Part model, mm, in its own coordinate system. A direction names the side the tool comes from. Coordinates: 2 decimals unless noted, no trailing zeros. Order: outer loops, then holes, each group sorted by start corner. A loop starts at its lowest first (then second) coordinate and runs counter-clockwise, first axis right, second up. Notation, with made-up numbers: M -13,65 L -2,65 A20 ccw -2,78 Z; hole C 87.25,37.25 d2. An arc over 180 degrees is marked long. Write item = value, one per line. Start each with the question number.
from build123d import *

# Parameters (mm, degrees)
SKETCH_1_W          = 23
SKETCH_1_H          = 23
EXTRUDE_1_DEPTH     = 1.6
SKETCH_2_W          = 5
SKETCH_2_H          = 4
EXTRUDE_2_DEPTH     = 1.6
FILLET_1_R          = 4
CUT_EXTRUDE_1_REACH = 18.575
SKETCH_3_R          = 1.6


with BuildPart() as part:
    # 草图1 → 凸台-拉伸1 (new body)
    with BuildSketch(Plane(origin=(0, 0, 0), x_dir=(1, 0, 0), z_dir=(0, 1, 0))):
        Rectangle(SKETCH_1_W, SKETCH_1_H)
    extrude(amount=EXTRUDE_1_DEPTH)

    # 草图2 → 凸台-拉伸2 (add)
    with BuildSketch(Plane(origin=(0, 1.6, 0), x_dir=(1, 0, 0), z_dir=(0, 1, 0))):
        Rectangle(SKETCH_2_W, SKETCH_2_H)
    extrude(amount=EXTRUDE_2_DEPTH)

    # 圆角1
    fillet_1_edges = [part.edges().sort_by_distance(p)[0] for p in [
        (11.5, 0.8, 11.5),
        (-11.5, 0.8, 11.5),
        (-11.5, 0.8, -11.5),
        (11.5, 0.8, -11.5),
    ]]
    fillet(fillet_1_edges, radius=FILLET_1_R)

    # 草图3 → 切除-拉伸1 (cut, up to next)
    with BuildSketch(Plane.XZ, mode=Mode.PRIVATE) as cut_extrude_1_sk1:
        with Locations(Location((-8, 8, 0), (0, 0, 270))):
            Circle(SKETCH_3_R)
    cut_extrude_1_tool1 = extrude(cut_extrude_1_sk1.sketch, amount=-CUT_EXTRUDE_1_REACH, mode=Mode.PRIVATE) & part.part
    # 草图3 → 切除-拉伸1 (cut, up to next)
    with BuildSketch(Plane.XZ, mode=Mode.PRIVATE) as cut_extrude_1_sk2:
        with Locations(Location((8, 8, 0), (0, 0, 270))):
            Circle(SKETCH_3_R)
    cut_extrude_1_tool2 = extrude(cut_extrude_1_sk2.sketch, amount=-CUT_EXTRUDE_1_REACH, mode=Mode.PRIVATE) & part.part
    # 草图3 → 切除-拉伸1 (cut, up to next)
    with BuildSketch(Plane.XZ, mode=Mode.PRIVATE) as cut_extrude_1_sk3:
        with Locations(Location((8, -8, 0), (0, 0, 270))):
            Circle(SKETCH_3_R)
    cut_extrude_1_tool3 = extrude(cut_extrude_1_sk3.sketch, amount=-CUT_EXTRUDE_1_REACH, mode=Mode.PRIVATE) & part.part
    # 草图3 → 切除-拉伸1 (cut, up to next)
    with BuildSketch(Plane.XZ, mode=Mode.PRIVATE) as cut_extrude_1_sk4:
        with Locations(Location((-8, -8, 0), (0, 0, 270))):
            Circle(SKETCH_3_R)
    cut_extrude_1_tool4 = extrude(cut_extrude_1_sk4.sketch, amount=-CUT_EXTRUDE_1_REACH, mode=Mode.PRIVATE) & part.part
    add(cut_extrude_1_tool1.solids().sort_by_distance((-8, 0, 8))[0], mode=Mode.SUBTRACT)
    add(cut_extrude_1_tool2.solids().sort_by_distance((8, 0, 8))[0], mode=Mode.SUBTRACT)
    add(cut_extrude_1_tool3.solids().sort_by_distance((8, 0, -8))[0], mode=Mode.SUBTRACT)
    add(cut_extrude_1_tool4.solids().sort_by_distance((-8, 0, -8))[0], mode=Mode.SUBTRACT)


solid = part.part
Item 1: Flat gauge pins, fed straight in: pin 1 (4 mm diameter, centred on x = -8, z = 8, fed in from +Y); pin 2 (2.5 mm diameter, centred on x = -8, z = -8, fed in from +Y); pin 3 (0.5 mm diameter, centred on x = 0, y = 3, fed in from -Z); pin 4 (0.5 mm diameter, centred on y = 2.5, z = 0, fed in from -X). Where does each tip first touch, or does it go through?
Item 2: Cut at B-B, the plane z = -8. Write the cut outline in (x, y).
Item 3: Wall check: line 1 along X through (y, z) = (0.4, -8); line 2 along Y through (x, z) = (1.5, -10); line 3 along X through (y, z) = (2.45, 0.5). Give the ranges that are in metal, low to high. Write a range as [from, to].
Item 4: Cut at C-C, the plane x = -1.5. Write the cut outline in (y, z), and give its area (3 significant figures).
Item 5: Cut at D-D, the plane x = -8. Write the cut outline in (y, z).
Item 6: Pull direction X, two halves, no side cores. Call faces 1 (the flat face through (-0.2, 1.6, 2.4)), 2 (the cylindrical face through (7.03, 0.79, 9.27)), 3 (the cylindrical face through (10.297, 0.811, -10.359)): pulls with the +X half, pulls with the -X half, needs draft (parallel to the pull), parting line crosses it, or undercut.
Item 7: 3-axis set-ups, long thin cutter, end or side, ignore diameter. For faces 4 (the flat face through (0, 2, 2)), 5 (the flat face through (2.5, 2, 0)), 6 (the flat face through (-2.5, 2, 0)): which of +Z, -Z, +X, -X, +Y, -Y reach the whole face in a straight line?
Item 8: Cut at A-A, the plane y = 0.3. Write the cut outline in (x, z), and give its area (3 significant figures).
Filled sheet:
q1.pin_1 = 1.6
q1.pin_2 = through
q1.pin_3 = -2
q1.pin_4 = -2.5
q2.outline = M -11.47,0 L -9.6,0 L -9.6,1.6 L -11.47,1.6 Z; M -6.4,0 L 6.4,0 L 6.4,1.6 L -6.4,1.6 Z; M 9.6,0 L 11.47,0 L 11.47,1.6 L 9.6,1.6 Z
q3.line_1 = [-11.47, -9.6], [-6.4, 6.4], [9.6, 11.47]
q3.line_2 = [0, 1.6]
q3.line_3 = [-2.5, 2.5]
q4.outline = M 0,-11.5 L 1.6,-11.5 L 1.6,-2 L 3.2,-2 L 3.2,2 L 1.6,2 L 1.6,11.5 L 0,11.5 Z
q4.area = 43.2 mm2
q5.outline = M 0,-11.47 L 1.6,-11.47 L 1.6,-9.6 L 0,-9.6 Z; M 0,-6.4 L 1.6,-6.4 L 1.6,6.4 L 0,6.4 Z; M 0,9.6 L 1.6,9.6 L 1.6,11.47 L 0,11.47 Z
q6.face_1 = needs draft
q6.face_2 = undercut
q6.face_3 = pulls with the +X half
q7.face_4 = +Z, +X, -X, +Y
q7.face_5 = +Z, -Z, +X, +Y
q7.face_6 = +Z, -Z, -X, +Y
q8.outline = M -11.5,-7.5 A4 ccw -7.5,-11.5 L 7.5,-11.5 A4 ccw 11.5,-7.5 L 11.5,7.5 A4 ccw 7.5,11.5 L -7.5,11.5 A4 ccw -11.5,7.5 Z; hole C -8,-8 d3.2; hole C -8,8 d3.2; hole C 8,-8 d3.2; hole C 8,8 d3.2
q8.area = 483 mm2
